The model under review builds one solid part; all positions refer to its coordinate system, in mm. Face numbers are marked on the shaded views. A direction names the side the tool comes from. Round coordinates to 2 decimals unless told otherwise and drop trailing zeros. Loops run counter-clockwise (first coordinate to the right, second up) from the corner with the lowest first, then second, coordinate; pieces in that order, holes last. Notation, with made-up numbers: M 82,-21 L 138,-21 A20 cw 138,-13 Z; hole C 35,43.5 d8. An arc over 180 degrees is marked long. Return JSON: item names as keys, results as strings. Group by question number.
Q1. Consider section C-C (y = 11). State the section outline as (x, z) points.
Q2. For the marked faces 1 and 2, list the 3-axis set-ups (+Z, -Z, +X, -X, +Y, -Y) from which the entire face can be reached by the end or side of a thin tool; tool diameter is ignored.
Q3. To check wall thickness, follow line 1 along Z through (x, y) = (5, 0); line 2 along Y through (x, z) = (6, -175); line 3 along Y through (x, z) = (3, -175). State the ranges of each line that lie inside material, in increasing order.
Q4. Consider section B-B (x = 0). State the section outline as (y, z) points, and give its area (3 significant figures).
Q5. Consider section A-A (y = 0). State the section outline as (x, z) points, and give its area (3 significant figures).
Q6. Clearance check with flat-ended pins moving along their axes: pin 1 Ø2 at (x, z) = (-2, -44.5) entering from -Y; pin 2 Ø5 at (x, z) = (16, -87) entering from +Y; pin 3 Ø10 at (x, y) = (-19.5, -19) entering from -Z. State where each tip first meets the part, or that it passes through.
Q7. Consider section D-D (z = -175). State the section outline as (x, y) points.
from build123d import *

# Parameters (mm, degrees)
SKETCH1_R           = 25
BOSS_EXTRUDE1_DEPTH = 10
SKETCH5_R           = 15
BOSS_EXTRUDE3_DEPTH = 185
SKETCH6_R           = 2.5
CUT_EXTRUDE1_DEPTH  = 92.5


with BuildPart() as part:
    # Sketch1 → Boss-Extrude1 (new body)
    with BuildSketch(Plane.XY):
        Circle(SKETCH1_R)
    extrude(amount=BOSS_EXTRUDE1_DEPTH)

    # Sketch5 → Boss-Extrude3 (add)
    with BuildSketch(Plane(origin=(0, 0, 0), x_dir=(-1, 0, 0), z_dir=(0, 0, -1))):
        Circle(SKETCH5_R)
    extrude(amount=BOSS_EXTRUDE3_DEPTH)

    # Sketch6 → Cut-Extrude1 (cut, symmetric)
    with BuildSketch(Plane(origin=(0, 0, 0), x_dir=(0, 0, -1), z_dir=(1, 0, 0))):
        with Locations((175, 0)):
            Circle(SKETCH6_R)
    extrude(amount=CUT_EXTRUDE1_DEPTH, both=True, mode=Mode.SUBTRACT)


solid = part.part
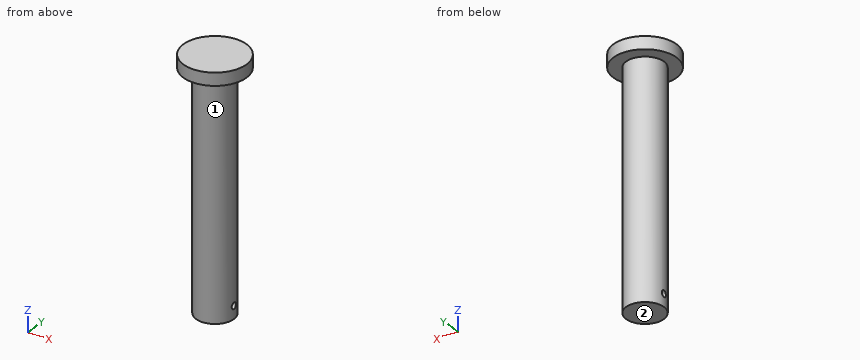
Values:
{
 "1": {"outline": "M -22.45,0 L -10.2,0 L -10.2,-185 L 10.2,-185 L 10.2,0 L 22.45,0 L 22.45,10 L -22.45,10 Z"},
 "2": {"face 1": "-Z", "face 2": "-Z, +X, -X, +Y, -Y"},
 "3": {"line 1": "z = -185 to -177.5, -172.5 to 10", "line 2": "y = -13.75 to -2.5, 2.5 to 13.75", "line 3": "y = -14.7 to -2.5, 2.5 to 14.7"},
 "4": {"outline": "M -25,0 L -15,0 L -15,-185 L 15,-185 L 15,0 L 25,0 L 25,10 L -25,10 Z; hole C 0,-175 d5", "area": "6,030 mm2"},
 "5": {"outline": "M -25,0 L -15,0 L -15,-172.5 L 15,-172.5 L 15,0 L 25,0 L 25,10 L -25,10 Z; M -15,-185 L 15,-185 L 15,-177.5 L -15,-177.5 Z", "area": "5,900 mm2"},
 "6": {"pin 1": "stops at y = -14.97", "pin 2": "stops at y = 6.54", "pin 3": "stops at z = 0"},
 "7": {"outline": "M -14.79,-2.5 A15 ccw 14.79,-2.5 Z; M -14.79,2.5 L 14.79,2.5 A15 ccw Z"}
}
